Check sheet for the drawn part. Datum: minimum x, y, z corner. Units: mm. A direction names the side the tool comes from. Give positions to 0.01 mm unless a question says otherwise; leave off trailing zeros. Order: outer loops, then holes, each group sorted by start corner. A loop starts at its lowest first (then second) coordinate and runs counter-clockwise, first axis right, second up. Notation, with made-up numbers: (76.5, 6) - (121.5, 6) arc R29 cw to (121.5, 32) - close; hole circle Ø7 at (74, 54). An arc over 180 degrees is marked (long way). Answer as a JSON object with one key per item and string values. Group by question number.
(1) Access from +Z, -Z, +X, -X, +Y, -Y to the whole of each face (thin tool, end or side, straight path). Record for the marked faces 4, 5, 6, 7 and 8.
(2) Section check A-A (x = 88.5). Record the boundary of the cut face in (y, z).
(3) Depth check by flat-ended pin: pin 1 Ø3 at (x, y) = (74.5, 102) entering from +Z; pin 2 Ø2 at (y, z) = (45, 11.5) entering from -X; pin 3 Ø1.3 at (y, z) = (114.5, 20) entering from +X; pin 4 Ø13.5 at (x, z) = (57.15, 22.225) entering from -Y. Enter the tip coordinate at first touch or a pass-through.
(4) Thickness scan on line 1 (Y direction, x = 43, z = 33); line 2 (Y direction, x = 6, z = 23.5); line 3 (Y direction, x = 96.5, z = 14). Record the ranges inside material, lowest first.
(5) Mould release check, pull along Z, two halves, no side actions. Record for the marked faces 1, 2 and 3: +Z half, -Z half, draft (parallel to the pull), parting line (faces both ways), or undercut.
(6) Section check C-C (x = 57.15). Record the boundary of the cut face in (y, z).
(7) Section check D-D (z = 7). Record the boundary of the cut face in (x, y).
(8) Section check B-B (z = 16). Record the boundary of the cut face in (x, y), then the cut area to 3 significant figures.
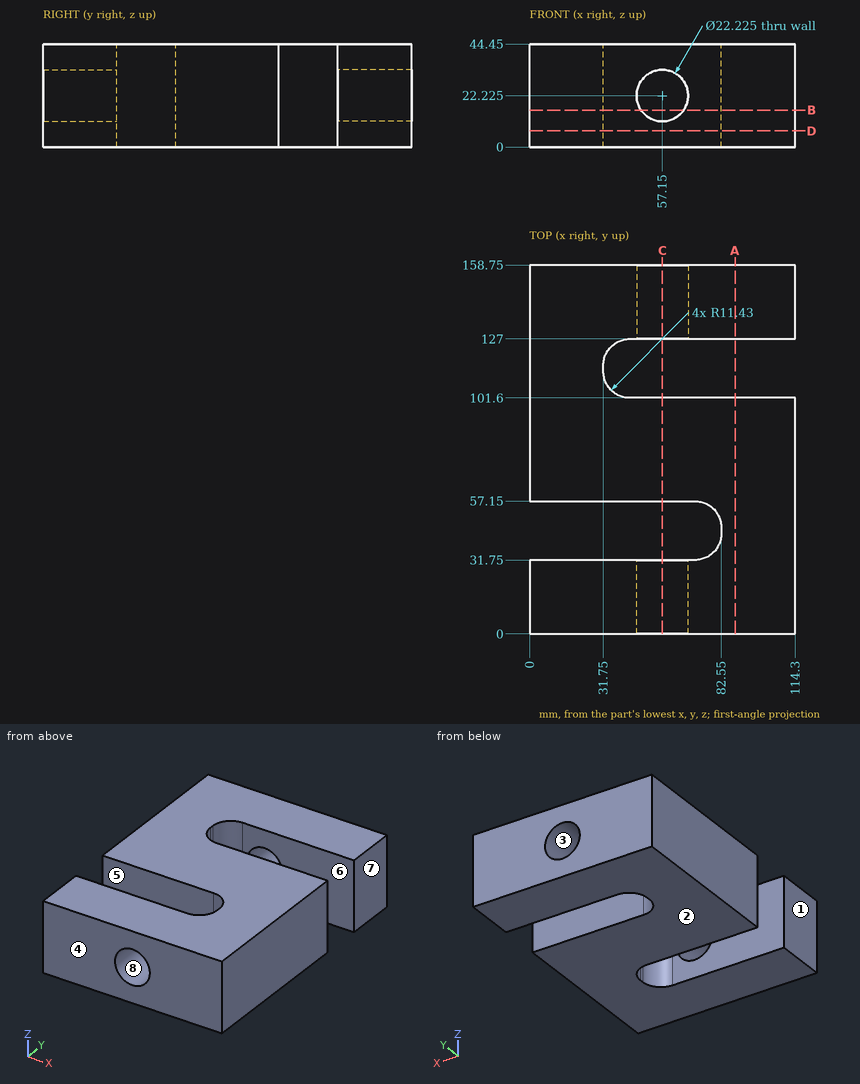
Solutions:
{
 "1": {"face 4": "+Z, -Z, +X, -X, -Y", "face 5": "+Z, -Z, -X", "face 6": "+Z, -Z, +X", "face 7": "+Z, -Z, +X, +Y, -Y", "face 8": "-Y"},
 "2": {"outline": "(0, 0) - (101.6, 0) - (101.6, 44.45) - (0, 44.45) - close; (127, 0) - (158.75, 0) - (158.75, 44.45) - (127, 44.45) - close"},
 "3": {"pin 1": "stops at z = 44.45", "pin 2": "stops at x = 82.55", "pin 3": "stops at x = 31.75", "pin 4": "stops at y = 57.15"},
 "4": {"line 1": "y = 0 to 31.75, 57.15 to 101.6, 127 to 158.75", "line 2": "y = 0 to 31.75, 57.15 to 158.75", "line 3": "y = 0 to 101.6, 127 to 158.75"},
 "5": {"face 1": "draft", "face 2": "-Z half", "face 3": "undercut"},
 "6": {"outline": "(0, 0) - (31.75, 0) - (31.75, 11.11) - (0, 11.11) - close; (0, 33.34) - (31.75, 33.34) - (31.75, 44.45) - (0, 44.45) - close; (57.15, 0) - (101.6, 0) - (101.6, 44.45) - (57.15, 44.45) - close; (127, 0) - (158.75, 0) - (158.75, 11.11) - (127, 11.11) - close; (127, 33.34) - (158.75, 33.34) - (158.75, 44.45) - (127, 44.45) - close"},
 "7": {"outline": "(0, 0) - (114.3, 0) - (114.3, 101.6) - (43.18, 101.6) arc R11.43 cw to (31.75, 113.03) - (31.75, 115.57) arc R11.43 cw to (43.18, 127) - (114.3, 127) - (114.3, 158.75) - (0, 158.75) - (0, 57.15) - (71.12, 57.15) arc R11.43 cw to (82.55, 45.72) - (82.55, 43.18) arc R11.43 cw to (71.12, 31.75) - (0, 31.75) - close"},
 "8": {"outline": "(0, 0) - (47.94, 0) - (47.94, 31.75) - (0, 31.75) - close; (0, 57.15) - (71.12, 57.15) arc R11.43 cw to (82.55, 45.72) - (82.55, 43.18) arc R11.43 cw to (71.12, 31.75) - (66.36, 31.75) - (66.36, 0) - (114.3, 0) - (114.3, 101.6) - (43.18, 101.6) arc R11.43 cw to (31.75, 113.03) - (31.75, 115.57) arc R11.43 cw to (43.18, 127) - (47.94, 127) - (47.94, 158.75) - (0, 158.75) - close; (66.36, 127) - (114.3, 127) - (114.3, 158.75) - (66.36, 158.75) - close", "area": "12,900 mm2"}
}
